from build123d import *

# Parameters (mm, degrees)
SKETCH_1_W          = 640
SKETCH_1_H          = 595
EXTRUDE_1_DEPTH     = 15
SKETCH_2_R          = 2.5
CUT_EXTRUDE_1_DEPTH = 16
SKETCH_2_3_R        = 2.5
CUT_EXTRUDE_2_DEPTH = 16
SKETCH_3_R          = 50
CUT_EXTRUDE_3_DEPTH = 16


with BuildPart() as part:
    # ｽｹｯﾁ1 → ﾎﾞｽ - 押し出し1 (new body)
    with BuildSketch(Plane.XY):
        Rectangle(SKETCH_1_W, SKETCH_1_H)
    extrude(amount=EXTRUDE_1_DEPTH)

    # ｽｹｯﾁ2 → ｶｯﾄ - 押し出し1 (cut, through all)
    with BuildSketch(Plane.XY.offset(15)):
        with Locations((-160, 287.5)):
            Circle(SKETCH_2_R)
        with Locations((0, 287.5)):
            Circle(SKETCH_2_R)
        with Locations((160, 287.5)):
            Circle(SKETCH_2_R)
    cut_extrude_1 = extrude(amount=-CUT_EXTRUDE_1_DEPTH, mode=Mode.SUBTRACT)

    # ｽｹｯﾁ2<3> → ｶｯﾄ - 押し出し2 (cut, through all)
    with BuildSketch(Plane.XY.offset(15)):
        with Locations((-295, 147.5)):
            Circle(SKETCH_2_3_R)
        with Locations((-295, -2.5)):
            Circle(SKETCH_2_3_R)
        with Locations((-295, -152.5)):
            Circle(SKETCH_2_3_R)
    cut_extrude_2 = extrude(amount=-CUT_EXTRUDE_2_DEPTH, mode=Mode.SUBTRACT)

    # ﾐﾗｰ1: ｶｯﾄ - 押し出し1 across plane
    add(cut_extrude_1.mirror(Plane.ZX), mode=Mode.SUBTRACT)

    # ﾐﾗｰ2: ｶｯﾄ - 押し出し2 across plane
    add(cut_extrude_2.mirror(Plane(origin=(0, 0, 0), x_dir=(0, 0, 1), z_dir=(1, 0, 0))), mode=Mode.SUBTRACT)

    # ｽｹｯﾁ3 → ｶｯﾄ - 押し出し3 (cut, through all)
    with BuildSketch(Plane.XY.offset(15)):
        with Locations((200, -200)):
            Circle(SKETCH_3_R)
    extrude(amount=-CUT_EXTRUDE_3_DEPTH, mode=Mode.SUBTRACT)


solid = part.part
Can you work these out from the model? Positions are in its coordinate system, mm. Give positions to 0.01 mm unless a question says otherwise; leave off trailing zeros. Loops run counter-clockwise (first coordinate to the right, second up) from the corner with the lowest first, then second, coordinate; pieces in that order, holes last. Notation, with made-up numbers: (27.5, 58.5) - (60.5, 58.5) arc R7 cw to (60.5, 65.5) - close; hole circle Ø5 at (-1, 47.5). An arc over 180 degrees is marked (long way). Return JSON: item names as keys, results as strings.
1. We'd pull the mould along X, two halves only. Please class faces 1 (the face through (160, -230, 8)), 2 (the face through (320, -4, 7)), 3 (the face through (-4, -297.5, 7)): +X half, -X half, draft (parallel to the pull), parting line (faces both ways), or undercut.
Output values:
{"face 1": "undercut", "face 2": "+X half", "face 3": "draft"}
2. I'm going to push a flat-ended pin straight in: pin 1 Ø3 at (x, y) = (-160, 287.5) entering from -Z. Where does the tip first touch, or does it pass through?
Output values:
{"pin 1": "passes through"}
3. I want a section at B-B on z = 7. Give the number of separate pieces and of enclosed holes in the cut face, and give its area (3 significant figures).
Output values:
{"separate pieces": "1", "enclosed holes": "13", "area": "373,000 mm²"}
4. I want a section at C-C on x = 230. Please give me the cut outline in (y, z), and give its area (4 significant figures).
Output values:
{"outline": "(-297.5, 0) - (-240, 0) - (-240, 15) - (-297.5, 15) - close; (-160, 0) - (297.5, 0) - (297.5, 15) - (-160, 15) - close", "area": "7,725 mm²"}
5. I want a section at A-A on y = -200. Please give me the cut outline in (x, z), and give its area (3 significant figures).
Output values:
{"outline": "(-320, 0) - (150, 0) - (150, 15) - (-320, 15) - close; (250, 0) - (320, 0) - (320, 15) - (250, 15) - close", "area": "8,100 mm²"}
6. If I drill on line 1 (Y direction, x = -295, z = 5.75); line 2 (X direction, y = 287.5, z = 6); line 3 (Y direction, x = -160, z = 7.5), over which ranges is the centre line in solid material (lowest first)?
Output values:
{"line 1": "y = -297.5 to -155, -150 to -5, 0 to 145, 150 to 297.5", "line 2": "x = -320 to -162.5, -157.5 to -2.5, 2.5 to 157.5, 162.5 to 320", "line 3": "y = -297.5 to -290, -285 to 285, 290 to 297.5"}
